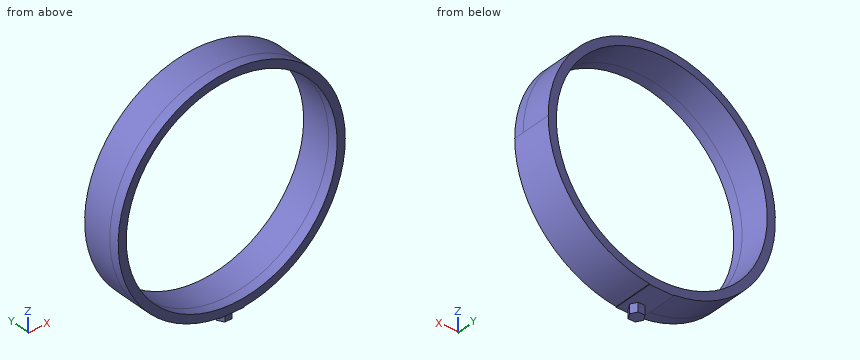
from build123d import *

# Parameters (mm, degrees)
F1_DEPTH      = 15
F1_DEPTH_BACK = 5
F2_DEPTH      = 5
F2_DEPTH_BACK = 15
F4_DEPTH      = 4.5


with BuildPart() as f1:
    # F0 (on Front) → F1 (new body, two sides)
    with BuildSketch(Plane.XZ) as f1_sk:
        with BuildLine():
            Line((-6, -52), (0, -52))
            Line((0, -52), (6, -52))
            Line((6, -52), (6, -55.6776436283))
            ThreePointArc((6, -55.6776436283), (41.665333312, -37.4165738677), (56, 0))
            ThreePointArc((56, 0), (-37.4165738677, 41.665333312), (-6, -55.6776436283))
            Line((-6, -55.6776436283), (-6, -52))
        make_face()
        with BuildLine():
            ThreePointArc((0, -52), (-36.7695526217, 36.7695526217), (52, 0))
            ThreePointArc((52, 0), (36.7695526217, -36.7695526217), (0, -52))
        make_face(mode=Mode.SUBTRACT)
        with BuildLine():
            Line((6, -52), (0, -52))
            Line((0, -52), (-6, -52))
            Line((-6, -52), (-6, -55.6776436283))
            ThreePointArc((-6, -55.6776436283), (-3.0043266147, -55.919352836), (0, -56))
            ThreePointArc((0, -56), (3.0043266147, -55.919352836), (6, -55.6776436283))
            Line((6, -55.6776436283), (6, -52))
        make_face()
    extrude(amount=-F1_DEPTH)
    extrude(f1_sk.sketch, amount=F1_DEPTH_BACK)

    # F0 (on Front) → F2 (join, two sides)
    with BuildSketch(Plane.XZ) as f2_sk:
        with BuildLine():
            Line((6, -56), (6, -55.6776436283))
            ThreePointArc((6, -55.6776436283), (3.0043266147, -55.919352836), (0, -56))
            Line((0, -56), (6, -56))
        make_face()
        with BuildLine():
            ThreePointArc((0, -56), (-3.0043266147, -55.919352836), (-6, -55.6776436283))
            Line((-6, -55.6776436283), (-6, -56))
            Line((-6, -56), (0, -56))
        make_face()
    extrude(amount=F2_DEPTH)
    extrude(f2_sk.sketch, amount=-F2_DEPTH_BACK)

    # F3 (on face) → F4 (join)
    with BuildSketch(Plane(origin=(0, 0, -56), x_dir=(1, 0, 0), z_dir=(0, 0, -1))):
        Polygon((-1.7145, 2.9696011096), (-3.429, 0), (-1.7145, -2.9696011096), (1.7145, -2.9696011096), (3.429, 0), (1.7145, 2.9696011096), align=None)
    extrude(amount=F4_DEPTH)


solid = f1.part
Here's how the part is built. I have some questions about the finished solid (model axes, mm). Round coordinates to 2 decimals unless told otherwise and drop trailing zeros. Write each loop counter-clockwise with the first axis right and the second up, starting at its lowest first coordinate (ties: lowest second). Pieces come first, ordered by that corner, then holes. Notation, with made-up numbers: (-26.5, 28.25) -> (-5.5, 28.25) arc R17 ccw to (-5.5, 59.25) -> close; hole circle Ø10 at (80, 85). An arc over 180 degrees is marked (long way). One line per item, written item: value.
1) If I drill on line 1 (X direction, y = -2, z = 0); line 2 (X direction, y = 1, z = 21); line 3 (Z direction, x = 42.5, y = 9.25), over which ranges is the centre line in solid material (lowest first)? Write a range as [from, to].
Filled sheet:
line 1: x = [-56, -52], [52, 56]
line 2: x = [-51.91, -47.57], [47.57, 51.91]
line 3: z = [-36.47, -29.96], [29.96, 36.47]
2) Suppose I cut it at D-D on x = -26.5. List the corners of the cut face in (y, z) for me.
Filled sheet:
outline: (-5, -49.33) -> (15, -49.33) -> (15, -44.74) -> (-5, -44.74) -> close; (-5, 44.74) -> (15, 44.74) -> (15, 49.33) -> (-5, 49.33) -> close
3) Suppose I cut it at C-C on y = 7.75. List the corners of the cut face in (x, z) for me.
Filled sheet:
outline: (-6, -56) -> (6, -56) -> (6, -55.68) arc R56 ccw (long way) to (-6, -55.68) -> close; hole circle Ø104 at (0, 0)
4) I'm going to push flat-ended pins straight in: pin 1 Ø3 at (x, y) = (18.5, -2.5) entering from -Z; pin 2 Ø2.5 at (x, z) = (-0.5, -57.5) entering from +Y; pin 3 Ø12 at (x, y) = (-29.5, 0.5) entering from +Z; pin 4 Ø3 at (x, z) = (40.5, -43.5) entering from -Y. Where does each tip first touch, or does it pass through?
Filled sheet:
pin 1: stops at z = -53.36
pin 2: stops at y = 2.97
pin 3: stops at z = 50.83
pin 4: passes through
5) Suppose I cut it at A-A on x = 0. List the corners of the cut face in (y, z) for me, plus the area to 3 significant figures.
Filled sheet:
outline: (-5, -56) -> (-2.97, -56) -> (-2.97, -60.5) -> (2.97, -60.5) -> (2.97, -56) -> (15, -56) -> (15, -52) -> (-5, -52) -> close; (-5, 52) -> (15, 52) -> (15, 56) -> (-5, 56) -> close
area: 187 mm2
6) Suppose I cut it at B-B on z = 18. List the corners of the cut face in (x, y) for me, plus the area to 3 significant figures.
Filled sheet:
outline: (-53.03, -5) -> (-48.79, -5) -> (-48.79, 15) -> (-53.03, 15) -> close; (48.79, -5) -> (53.03, -5) -> (53.03, 15) -> (48.79, 15) -> close
area: 170 mm2
